Geometry check sheet. Reference: the model listing, model coordinates, mm. A direction names the side the tool comes from. Round coordinates to 2 decimals unless told otherwise and drop trailing zeros. Order: outer loops, then holes, each group sorted by start corner. A loop starts at its lowest first (then second) coordinate and runs counter-clockwise, first axis right, second up.
(1) Sectioned sample at A-A (x = 0). Record the boundary of the cut face in (y, z).
(2) Set-up check for faces 4 (the face through (15, 36, -39)), 5 (the face through (0, 36.123, -20)), 6 (the face through (4, -3, -79)), 7 (the face through (0, 39.623, -39)), 8 (the face through (-30.5, -12.6, -38.5)): record each of +Z, -Z, +X, -X, +Y, -Y from which the full face is reachable in a straight line by a thin tool's end or side.
(3) Sectioned sample at C-C (z = -20). Record the boundary of the cut face in (x, y), plus the area to 3 significant figures.
(4) Sectioned sample at B-B (y = 0). Record the boundary of the cut face in (x, z).
(5) Go/stop test with flat-tipped pins: pin 1 (1.5 mm diameter, centred on x = -12, y = -24.5, fed in from +Z); pin 2 (12 mm diameter, centred on y = 6.5, z = -65.5, fed in from +X); pin 3 (2.5 mm diameter, centred on x = -1.5, z = -18, fed in from +Y); pin 4 (6 mm diameter, centred on x = 0, y = 0, fed in from -Z). Record where each tip stops, or that it passes through.
(6) Release check for a two-part mould opening along Y. For faces 1 (the face through (1.322, -34.975, -39.44)), 2 (the face through (0, -7, -78)), 3 (the face through (-15, 36, -39)) record: +Y half, -Y half, draft (parallel to the pull), parting line (faces both ways), or undercut.
(7) Sectioned sample at D-D (x = 20). Record the boundary of the cut face in (y, z).
(8) Material ranges on line 1 along Z through (x, y) = (0, 38.9); line 2 along X through (y, z) = (0, -79); line 3 along X through (y, z) = (38, -20), recorded low to high.
from build123d import *

# Parameters (mm, degrees)
PAD_DEPTH            = 80
SKETCH001_R          = 33
POCKET_DEPTH         = 78
SKETCH002_R          = 5
POCKET001_DEPTH      = 80.001
SKETCH003_R          = 4.5
POCKET002_DEPTH      = 3.5
LINEARPATTERN_COUNT  = 2
LINEARPATTERN_PITCH  = 40
BODY_PLACEMENT_ANGLE = 180


with BuildPart() as part:
    # Sketch → Pad (new body)
    with BuildSketch(Plane.XY):
        with BuildLine():
            Line((-15, 39.622777), (15, 39.622777))
            Line((15, 39.622777), (15, 31.622777))
            ThreePointArc((-15, 31.622777), (0, -35), (15, 31.622777))
            Line((-15, 39.622777), (-15, 31.622777))
        make_face()
    extrude(amount=PAD_DEPTH)

    # Sketch001 → Pocket (cut)
    with BuildSketch(Plane.XY):
        Circle(SKETCH001_R)
    extrude(amount=POCKET_DEPTH, mode=Mode.SUBTRACT)

    # Sketch002 → Pocket001 (cut, through all)
    with BuildSketch(Plane.XY):
        Circle(SKETCH002_R)
    extrude(amount=POCKET001_DEPTH, mode=Mode.SUBTRACT)

    # Sketch003 (on Face1 of Pocket001) → Pocket002 (cut)
    with BuildSketch(Plane(origin=(0, 39.622777, 0), x_dir=(-1, 0, 0), z_dir=(0, 1, 0))):
        with Locations((0, 20)):
            Circle(SKETCH003_R)
    pocket002 = extrude(amount=-POCKET002_DEPTH, mode=Mode.SUBTRACT)

    # LinearPattern: Pocket002 ×2
    with Locations(*[(0, 0, i * LINEARPATTERN_PITCH) for i in range(1, LINEARPATTERN_COUNT)]):
        add(pocket002, mode=Mode.SUBTRACT)


with BuildPart() as part_1:
    # Body placement: moved
    add(part.part.rotate(Axis((0, 0, 0), (0, 1, 0)), BODY_PLACEMENT_ANGLE))


solid = part_1.part
Answer below:
1. outline: (-35, -80) - (-5, -80) - (-5, -78) - (-33, -78) - (-33, 0) - (-35, 0) - close; (5, -80) - (39.62, -80) - (39.62, -64.5) - (36.12, -64.5) - (36.12, -55.5) - (39.62, -55.5) - (39.62, -24.5) - (36.12, -24.5) - (36.12, -15.5) - (39.62, -15.5) - (39.62, 0) - (33, 0) - (33, -78) - (5, -78) - close
2. face 4: +Z, -Z, +X, +Y
2. face 5: +Y
2. face 6: +Z, -Z
2. face 7: +Z, -Z, +X, -X, +Y
2. face 8: +Z
3. outline: (-15, 31.62) arc R35 ccw (long way) to (15, 31.62) - (15, 39.62) - (4.5, 39.62) - (4.5, 36.12) - (-4.5, 36.12) - (-4.5, 39.62) - (-15, 39.62) - close; hole circle Ø66 at (0, 0)
3. area: 568 mm2
4. outline: (-35, -80) - (-5, -80) - (-5, -78) - (-33, -78) - (-33, 0) - (-35, 0) - close; (5, -80) - (35, -80) - (35, 0) - (33, 0) - (33, -78) - (5, -78) - close
5. pin 1: stops at z = -78
5. pin 2: stops at x = 35
5. pin 3: stops at y = 36.12
5. pin 4: passes through
6. face 1: parting line
6. face 2: undercut
6. face 3: draft
7. outline: (-28.72, -80) - (28.72, -80) - (28.72, 0) - (26.25, 0) - (26.25, -78) - (-26.25, -78) - (-26.25, 0) - (-28.72, 0) - close
8. line 1: z = -80 to -64.5, -55.5 to -24.5, -15.5 to 0
8. line 2: x = -35 to -5, 5 to 35
8. line 3: x = -15 to -4.5, 4.5 to 15
